from build123d import *

# Parameters (mm, degrees)
ESQUISSE1_R        = 20
BOSS_EXTRU_1_DEPTH = 10
CHANFREIN1_SIZE    = 1
ESQUISSE2_R        = 7
BOSS_EXTRU_2_DEPTH = 3
TROU_TARAUD_M101_D = 8.5


with BuildPart() as part:
    # Esquisse1 → Boss.-Extru.1 (new body)
    with BuildSketch(Plane.XY):
        Circle(ESQUISSE1_R)
    extrude(amount=BOSS_EXTRU_1_DEPTH)

    # Chanfrein1
    chanfrein1_edges = [part.edges().sort_by_distance(p)[0] for p in [
        (-20, 0, 0),
        (-20, 0, 10),
    ]]
    chamfer(chanfrein1_edges, length=CHANFREIN1_SIZE)

    # Esquisse2 → Boss.-Extru.2 (add)
    with BuildSketch(Plane.XY.offset(10)):
        Circle(ESQUISSE2_R)
    extrude(amount=BOSS_EXTRU_2_DEPTH)

    # Trou taraudé M101 (through all)
    with Locations(Plane.XY.offset(13)):
        with Locations((0, 0)):
            Hole(TROU_TARAUD_M101_D / 2)


solid = part.part
Read the model definition and answer for the solid it produces. Units are mm, in the model's axes. Coordinates: 2 decimals unless noted, no trailing zeros. Order: outer loops, then holes, each group sorted by start corner. A loop starts at its lowest first (then second) coordinate and runs counter-clockwise, first axis right, second up. Notation, with made-up numbers: (5, -3.5) - (18, -3.5) arc R21 ccw to (18, 22.5) - close; hole circle Ø11 at (46.25, 24.5). An arc over 180 degrees is marked (long way). Use one line per item in the form item = value.
(1) Section A-A, the plane y = 0 is taken. Give the vertices of the cut face in (x, z).
Computed values:
outline = (-20, 1) - (-19, 0) - (-4.25, 0) - (-4.25, 13) - (-7, 13) - (-7, 10) - (-19, 10) - (-20, 9) - close; (4.25, 0) - (19, 0) - (20, 1) - (20, 9) - (19, 10) - (7, 10) - (7, 13) - (4.25, 13) - close
(2) Section C-C, the plane z = 8.5 is taken. Give the vertices of the cut face in (x, y).
Computed values:
outline = circle Ø40 at (0, 0); hole circle Ø8.5 at (0, 0)
(3) Given pin 1 Ø2 at (x, z) = (-14, 7.5) entering from -Y; pin 2 Ø6 at (x, z) = (-14, 3.5) entering from +Y; pin 3 Ø1 at (y, z) = (-13, 1.5) entering from -X, each flat-ended and moving along its own axis, determine where each tip first touches the part or whether it passes through.
Computed values:
pin_1 = -15.2
pin_2 = 16.7
pin_3 = -15.61
(4) For a pull along Y with two mould halves and no side action, classify faces 1 (the face through (6.466, -2.681, 11.479)), 2 (the face through (-2.285, 3.584, 6.409)), 3 (the face through (8, 0, 10)) as pulls with the +Y half, pulls with the -Y half, needs draft (parallel to the pull), parting line crosses it, or undercut.
Computed values:
face_1 = parting line crosses it
face_2 = undercut
face_3 = needs draft
(5) Straight lines are drawn through the part: L1, parallel to Y at x = 0, z = 8; L2, parallel to Z at x = 8.5, y = 11.5; L3, parallel to Y at x = 3, z = 4.5. For each, find the intervals that lie inside material, in ascending order.
Computed values:
L1 = -20 to -4.25, 4.25 to 20
L2 = 0 to 10
L3 = -19.77 to -3.01, 3.01 to 19.77
